Build history of the part. All positions in model axes, mm. Round coordinates to 2 decimals unless told otherwise and drop trailing zeros. Loops run counter-clockwise (first coordinate to the right, second up) from the corner with the lowest first, then second, coordinate; pieces in that order, holes last.
from build123d import *

# Parameters (mm, degrees)
F0_W     = 137.7488821745
F0_H     = 67.785397172
F2_DEPTH = 19.75811
F1_W     = 137.6349329948
F1_H     = 94.5436730981
F3_DEPTH = 41.69879
F5_D     = 17.78


with BuildPart() as f2:
    # F0 (on Top) → F2 (new body)
    with BuildSketch(Plane.XY):
        Rectangle(F0_W, F0_H)
    extrude(amount=F2_DEPTH)

    # F1 (on Front) → F3 (join)
    with BuildSketch(Plane.XZ):
        with Locations((0.1108199358, 47.271836549)):
            Rectangle(F1_W, F1_H)
    extrude(amount=F3_DEPTH)

    # F5 (through all)
    with Locations(Plane(origin=(0, 0, 0), x_dir=(1, 0, 0), z_dir=(0, 1, 0))):
        with Locations((-36.0051579773, -46.4185513556), (36.2534709275, -45.9219291806)):
            Hole(F5_D / 2)


solid = f2.part
(1) Slice it at D-D on x = 3.5. List the corners of the cut face in (y, z), plus the area to 3 significant figures.
Responses:
outline: (-41.7, 0) - (33.89, 0) - (33.89, 19.76) - (0, 19.76) - (0, 94.54) - (-41.7, 94.54) - close
area: 4,610 mm2
(2) Pull direction Z, two halves, no side cores. Call faces 1 (the face through (-34.1, -21.1, 55.1)), 2 (the face through (68.928, -21, 47)), 3 (the face through (-1, -21, 94.544)): +Z half, -Z half, draft (parallel to the pull), parting line (faces both ways), or undercut.
Responses:
face 1: undercut
face 2: draft
face 3: +Z half
(3) Slice it at B-B on y = -1.5. List the corners of the cut face in (x, z), plus the area to 3 significant figures.
Responses:
outline: (-68.87, 0) - (68.93, 0) - (68.93, 94.54) - (-68.71, 94.54) - (-68.71, 19.76) - (-68.87, 19.76) - close; hole circle Ø17.78 at (-36.01, 46.42); hole circle Ø17.78 at (36.25, 45.92)
area: 12,500 mm2
(4) Slice it at C-C on z = 25. List the corners of the cut face in (x, y), plus the area to 3 significant figures.
Responses:
outline: (-68.71, -41.7) - (68.93, -41.7) - (68.93, 0) - (-68.71, 0) - close
area: 5,740 mm2
(5) Probe line 1 (X direction, y = -35.5, z = 46); line 2 (Z direction, x = 19, y = 20); line 3 (X direction, y = -24.5, z = 44). List the from-to ranges inside material, lowest first.
Responses:
line 1: x = -68.71 to -44.89, -27.13 to 27.36, 45.14 to 68.93
line 2: z = 0 to 19.76
line 3: x = -68.71 to -44.56, -27.45 to 27.57, 44.93 to 68.93
(6) Pin check, flat tips, straight feed: P1, Ø16, axis at x = 36.25, z = 45.92, coming from the +Y side; P2, Ø16, axis at y = 25.5, z = 10.5, coming from the +X side; P3, Ø1.5, axis at y = -20.5, z = 30.5, coming from the -X side; P4, Ø20.5, axis at x = -7.5, y = 12, coming from the +Z side. Stop position of each tip, or through.
Responses:
P1: passes through
P2: stops at x = 68.87
P3: stops at x = -68.71
P4: stops at z = 19.76
(7) Slice it at A-A on x = 36.5. List the corners of the cut face in (y, z).
Responses:
outline: (-41.7, 0) - (33.89, 0) - (33.89, 19.76) - (0, 19.76) - (0, 37.04) - (-41.7, 37.04) - close; (-41.7, 54.81) - (0, 54.81) - (0, 94.54) - (-41.7, 94.54) - close
